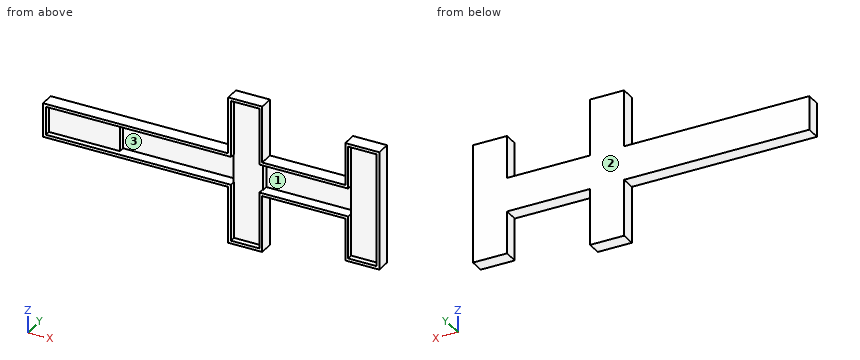
from build123d import *

# Parameters (mm, degrees)
SKETCH_3_W           = 10
SKETCH_3_H           = 40
SKETCH_3_W_2         = 31.25
SKETCH_3_H_2         = 10
SKETCH_3_W_3         = 40.25
SKETCH_3_W_4         = 25
EXTRUDE_1_DEPTH      = 1
EXTRUDE_2_DEPTH      = 4
EXTRUDE_2_DEPTH_BACK = 1
SKETCH_5_W           = 25
SKETCH_5_H           = 10
SKETCH_5_W_2         = 10
SKETCH_5_H_2         = 40
EXTRUDE_3_DEPTH      = 2


with BuildPart() as part:
    # 草图3 → 凸台-拉伸1 (new body)
    with BuildSketch(Plane(origin=(0, 0, 0), x_dir=(1, 0, 0), z_dir=(0, 1, 0))):
        with Locations((20.5, 0)):
            Rectangle(SKETCH_3_W, SKETCH_3_H)
        with Locations((-0.125, 0)):
            Rectangle(SKETCH_3_W_2, SKETCH_3_H_2)
        Polygon((-15.75, -5), (-15.75, 5), (-15.75, 25), (-25.75, 25), (-25.75, 5), (-25.75, -5), (-25.75, -25), (-15.75, -25), align=None)
        with Locations((-45.875, 0)):
            Rectangle(SKETCH_3_W_3, SKETCH_3_H_2)
        with Locations((-78.5, 0)):
            Rectangle(SKETCH_3_W_4, SKETCH_3_H_2)
    extrude(amount=EXTRUDE_1_DEPTH)

    # 草图4 → 凸台-拉伸2 (add, two sides)
    with BuildSketch(Plane.XZ) as extrude_2_sk:
        Polygon((14.5, -21), (26.5, -21), (26.5, 21), (14.5, 21), (14.5, 6), (-14.75, 6), (-14.75, 26), (-26.75, 26), (-26.75, 6), (-92, 6), (-92, -6), (-26.75, -6), (-26.75, -26), (-14.75, -26), (-14.75, -6), (14.5, -6), align=None)
        Polygon((15.5, -20), (25.5, -20), (25.5, 20), (15.5, 20), (15.5, 5), (-15.75, 5), (-15.75, 25), (-25.75, 25), (-25.75, 5), (-91, 5), (-91, -5), (-25.75, -5), (-25.75, -25), (-15.75, -25), (-15.75, -5), (15.5, -5), align=None, mode=Mode.SUBTRACT)
    extrude(amount=EXTRUDE_2_DEPTH)
    extrude(extrude_2_sk.sketch, amount=-EXTRUDE_2_DEPTH_BACK)

    # 草图5 → 凸台-拉伸3 (add)
    with BuildSketch(Plane.XZ):
        Polygon((-25.75, 25), (-25.75, 5), (-26, 5), (-26, -5), (-25.75, -5), (-25.75, -25), (-15.75, -25), (-15.75, -5), (-15.5, -5), (-15.5, 5), (-15.75, 5), (-15.75, 25), align=None)
        with Locations((-78.5, 0)):
            Rectangle(SKETCH_5_W, SKETCH_5_H)
        with Locations((20.5, 0)):
            Rectangle(SKETCH_5_W_2, SKETCH_5_H_2)
    extrude(amount=EXTRUDE_3_DEPTH)


solid = part.part
Geometry: final body of the model. Coordinates: model frame, mm. Face numbers are marked on the shaded views. Give positions to 0.01 mm unless a question says otherwise; leave off trailing zeros. Write each loop counter-clockwise with the first axis right and the second up, starting at its lowest first coordinate (ties: lowest second). Pieces come first, ordered by that corner, then holes. Notation, with made-up numbers: (-39, 19.5) - (3, 19.5) arc R22 ccw to (3, 50.5) - close; hole circle Ø4 at (-30.5, -30). An arc over 180 degrees is marked (long way). Return JSON: item names as keys, results as strings. Group by question number.
1) Section C-C on x = 9.5. Return the cut outline in (y, z), plus the area to 3 significant figures.
2) First-contact query: P1, Ø1.5, axis at y = -2.5, z = -13.5, coming from the -X side; P2, Ø2, axis at x = -77, y = -0.5, coming from the +Z side; P3, Ø2.5, axis at x = 1, y = -0.5, coming from the -Z side. Flat tips, straight axial feed; report the tip coordinate or a pass-through.
3) Line query: line 1 (X direction, y = -3.25, z = -8.5); line 2 (Z direction, x = -10, y = -1.05); line 3 (X direction, y = -0.25, z = 0.5). Output: solid intervals per line, ascending.
4) Section A-A on y = -1.05. Return the cut outline in (x, z).
5) Section B-B on z = 16.5. Return the cut outline in (x, y), plus the area to 3 significant figures.
6) Mould query, pull axis Z, two halves, no side actions, for the marked faces 1, 2 and 3. Classes: released by +Z, released by -Z, zero draft, split by the parting line, or undercut.
7) Section D-D on z = 3. Return the cut outline in (x, y).
Filled in:
{
 "1": {"outline": "(-4, -6) - (1, -6) - (1, 6) - (-4, 6) - (-4, 5) - (0, 5) - (0, -5) - (-4, -5) - close", "area": "20.0 mm^2"},
 "2": {"P1": "stops at x = -26.75", "P2": "stops at z = 6", "P3": "stops at z = -6"},
 "3": {"line 1": "x = -26.75 to -25.75, -15.75 to -14.75, 14.5 to 15.5, 25.5 to 26.5", "line 2": "z = -6 to -5, 5 to 6", "line 3": "x = -92 to -66, -26 to -15.5, 15.5 to 26.5"},
 "4": {"outline": "(-92, -6) - (-26.75, -6) - (-26.75, -26) - (-14.75, -26) - (-14.75, -6) - (14.5, -6) - (14.5, -21) - (26.5, -21) - (26.5, 21) - (14.5, 21) - (14.5, 6) - (-14.75, 6) - (-14.75, 26) - (-26.75, 26) - (-26.75, 6) - (-92, 6) - close; hole (-66, -5) - (-26, -5) - (-26, 5) - (-66, 5) - close; hole (-15.5, -5) - (15.5, -5) - (15.5, 5) - (-15.5, 5) - close"},
 "5": {"outline": "(-26.75, -4) - (-25.75, -4) - (-25.75, -2) - (-15.75, -2) - (-15.75, -4) - (-14.75, -4) - (-14.75, 1) - (-26.75, 1) - close; (14.5, -4) - (15.5, -4) - (15.5, -2) - (25.5, -2) - (25.5, -4) - (26.5, -4) - (26.5, 1) - (14.5, 1) - close", "area": "80.0 mm^2"},
 "6": {"face 1": "undercut", "face 2": "zero draft", "face 3": "undercut"},
 "7": {"outline": "(-92, -4) - (-91, -4) - (-91, -2) - (-66, -2) - (-66, 0) - (-26, 0) - (-26, -2) - (-15.5, -2) - (-15.5, 0) - (15.5, 0) - (15.5, -2) - (25.5, -2) - (25.5, -4) - (26.5, -4) - (26.5, 1) - (-92, 1) - close"}
}
